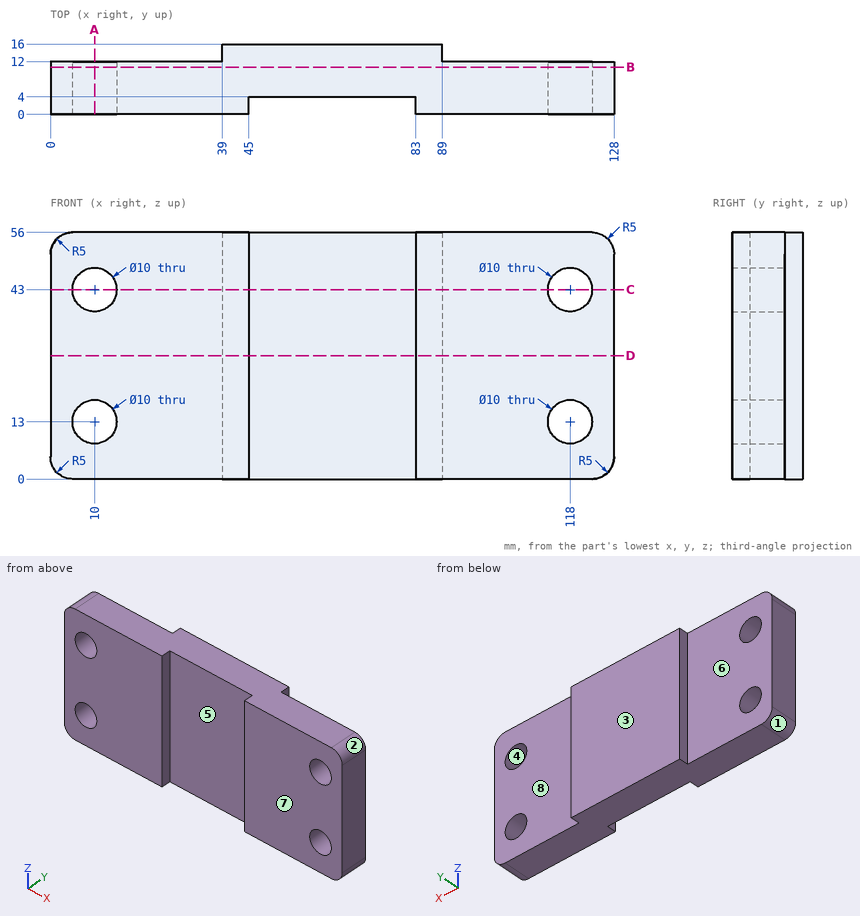
Geometry: see drawing. Coordinates: mm, zero at the bounding-box minimum. A direction names the side the tool comes from. Give positions to 0.01 mm unless a question says otherwise; leave off trailing zeros. Loops run counter-clockwise (first coordinate to the right, second up) from the corner with the lowest first, then second, coordinate; pieces in that order, holes last. Notation, with made-up numbers: (12, -26.5) - (53, -26.5) arc R25 cw to (53, 6.5) - close; hole circle Ø4 at (1, 55.25). An arc over 180 degrees is marked (long way). One line per question, with ' | ' between items. Start each with the question number.
(1) Pull-direction query (X, two-part tool) for the marked faces 1, 2, 3 and 4; classes: released by +X, released by -X, zero draft, split by the parting line, or undercut.
(2) Ray query, line 1 (Z direction, x = 10, y = 7.75); line 2 (X direction, y = 9.5, z = 43.5); line 3 (X direction, y = 1.75, z = 14.5). Return the intervals inside material, ascending. Write a range as from..to.
(3) Section query D-D on z = 28. Return loops of the section in (x, y), then the cut area to 3 significant figures.
(4) Section query B-B on y = 10.75. Return loops of the section in (x, z), then the cut area to 3 significant figures.
(5) Section query A-A on x = 10. Return loops of the section in (y, z), then the cut area to 3 significant figures.
(6) Section query C-C on z = 43. Return loops of the section in (x, y).
(7) Contact query for flat-ended pins moving along their axis: pin 1 (19 mm diameter, centred on x = 64, z = 18.5, fed in from -Y); pin 2 (8 mm diameter, centred on x = 10, z = 13, fed in from +Y); pin 3 (16 mm diameter, centred on x = 118, z = 13, fed in from +Y); pin 4 (4.5 mm diameter, centred on y = 14.5, z = 16, fed in from +X). Output: stop coordinate, or through.
(8) Reachability of the marked faces 5, 6, 7 and 8 from +Z, -Z, +X, -X, +Y, -Y: full face, straight path, thin tool, end or side. Return the list, or none.
The answers:
1) face 1: released by -X | face 2: released by +X | face 3: zero draft | face 4: undercut
2) line 1: 0..8, 18..38, 48..56 | line 2: 0..5.03, 14.97..113.03, 122.97..128 | line 3: 0..5.23, 14.77..45, 83..113.23, 122.77..128
3) outline: (0, 0) - (45, 0) - (45, 4) - (83, 4) - (83, 0) - (128, 0) - (128, 12) - (89, 12) - (89, 16) - (39, 16) - (39, 12) - (0, 12) - close | area: 1,580 mm2
4) outline: (0, 5) arc R5 ccw to (5, 0) - (123, 0) arc R5 ccw to (128, 5) - (128, 51) arc R5 ccw to (123, 56) - (5, 56) arc R5 ccw to (0, 51) - close; hole circle Ø10 at (10, 13); hole circle Ø10 at (10, 43); hole circle Ø10 at (118, 13); hole circle Ø10 at (118, 43) | area: 6,830 mm2
5) outline: (0, 0) - (12, 0) - (12, 8) - (0, 8) - close; (0, 18) - (12, 18) - (12, 38) - (0, 38) - close; (0, 48) - (12, 48) - (12, 56) - (0, 56) - close | area: 432 mm2
6) outline: (0, 0) - (5, 0) - (5, 12) - (0, 12) - close; (15, 0) - (45, 0) - (45, 4) - (83, 4) - (83, 0) - (113, 0) - (113, 12) - (89, 12) - (89, 16) - (39, 16) - (39, 12) - (15, 12) - close; (123, 0) - (128, 0) - (128, 12) - (123, 12) - close
7) pin 1: y = 4 | pin 2: through | pin 3: y = 12 | pin 4: x = 89
8) face 5: +Z, -Z, -Y | face 6: +Z, -Z, -X, +Y | face 7: +Z, -Z, +X, -X, -Y | face 8: +Z, -Z, +X, +Y
